Source: CAD feature listing. Evaluate the final solid. Frame: model axes, mm. Face numbers are marked on the shaded views. A direction names the side the tool comes from. Give positions to 0.01 mm unless a question says otherwise; leave off trailing zeros. Loops run counter-clockwise (first coordinate to the right, second up) from the corner with the lowest first, then second, coordinate; pieces in that order, holes last. Notation, with made-up numbers: M 83,22.25 L 102,22.25 A23 cw 102,59.25 Z; hole C 85,10.5 d5. An arc over 180 degrees is marked long. Answer in a Markdown table with one row per item.
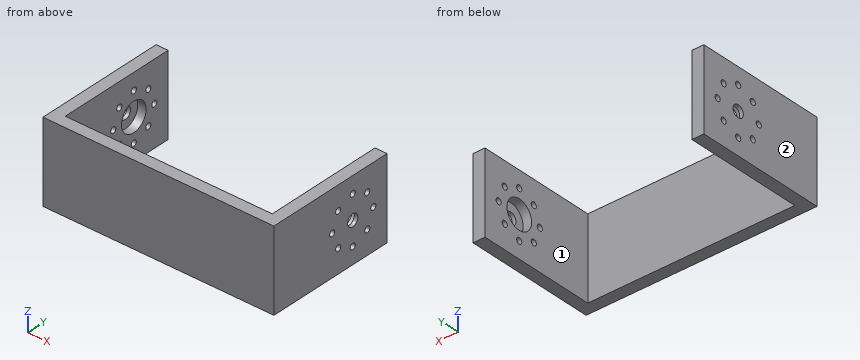
```python
from build123d import *

# Parameters (mm, degrees)
SKETCH1_W               = 57.8
SKETCH1_H               = 20.3
YAWMOUNT_DEPTH          = 3
SKETCH2_W               = 3
SKETCH2_H               = 20.3
BODYCONNECTORS_DEPTH    = 30
AXLE_MOUNTS_REACH       = 71.584
SKETCH3_R               = 1.5
SKETCH3_R_2             = 0.75
SKETCH4_R               = 3.6
SLIDE_COUNTERBORE_DEPTH = 2.12
GEAR_COUNTERBORE_START  = -2.1
SKETCH5_R               = 3.6
GEAR_COUNTERBORE_DEPTH  = 2.1


with BuildPart() as part:
    # Sketch1 → YawMount (new body)
    with BuildSketch(Plane(origin=(0, 0, 0), x_dir=(1, 0, 0), z_dir=(0, 1, 0))):
        with Locations((28.9, 10.15)):
            Rectangle(SKETCH1_W, SKETCH1_H)
    extrude(amount=YAWMOUNT_DEPTH)

    # Sketch2 → BodyConnectors (add)
    with BuildSketch(Plane(origin=(0, 3, 0), x_dir=(1, 0, 0), z_dir=(0, 1, 0))):
        with Locations((1.5, 10.15)):
            Rectangle(SKETCH2_W, SKETCH2_H)
        with Locations((56.3, 10.15)):
            Rectangle(SKETCH2_W, SKETCH2_H)
    extrude(amount=BODYCONNECTORS_DEPTH)

    # Axle-Mounts: up to this face of the body (flat: up to its plane)
    axle_mounts_end = Plane(part.part.faces().sort_by_distance((0, 16.5, -10.15))[0])
    # Sketch3 → Axle-Mounts (cut, up to the picked face)
    with BuildSketch(Plane(origin=(57.8, 0, 0), x_dir=(0, 0, -1), z_dir=(1, 0, 0)), mode=Mode.PRIVATE) as axle_mounts_sk1:
        with Locations((10.15, 23)):
            Circle(SKETCH3_R)
    axle_mounts_tool1 = split(extrude(axle_mounts_sk1.sketch, amount=-AXLE_MOUNTS_REACH, mode=Mode.PRIVATE), bisect_by=axle_mounts_end, keep=Keep.BOTH, mode=Mode.PRIVATE)
    # Sketch3 → Axle-Mounts (cut, up to the picked face)
    with BuildSketch(Plane(origin=(57.8, 0, 0), x_dir=(0, 0, -1), z_dir=(1, 0, 0)), mode=Mode.PRIVATE) as axle_mounts_sk2:
        with Locations((16.15, 23)):
            Circle(SKETCH3_R_2)
    axle_mounts_tool2 = split(extrude(axle_mounts_sk2.sketch, amount=-AXLE_MOUNTS_REACH, mode=Mode.PRIVATE), bisect_by=axle_mounts_end, keep=Keep.BOTH, mode=Mode.PRIVATE)
    # Sketch3 → Axle-Mounts (cut, up to the picked face)
    with BuildSketch(Plane(origin=(57.8, 0, 0), x_dir=(0, 0, -1), z_dir=(1, 0, 0)), mode=Mode.PRIVATE) as axle_mounts_sk3:
        with Locations((14.392640687, 18.757359313)):
            Circle(SKETCH3_R_2)
    axle_mounts_tool3 = split(extrude(axle_mounts_sk3.sketch, amount=-AXLE_MOUNTS_REACH, mode=Mode.PRIVATE), bisect_by=axle_mounts_end, keep=Keep.BOTH, mode=Mode.PRIVATE)
    # Sketch3 → Axle-Mounts (cut, up to the picked face)
    with BuildSketch(Plane(origin=(57.8, 0, 0), x_dir=(0, 0, -1), z_dir=(1, 0, 0)), mode=Mode.PRIVATE) as axle_mounts_sk4:
        with Locations((10.15, 17)):
            Circle(SKETCH3_R_2)
    axle_mounts_tool4 = split(extrude(axle_mounts_sk4.sketch, amount=-AXLE_MOUNTS_REACH, mode=Mode.PRIVATE), bisect_by=axle_mounts_end, keep=Keep.BOTH, mode=Mode.PRIVATE)
    # Sketch3 → Axle-Mounts (cut, up to the picked face)
    with BuildSketch(Plane(origin=(57.8, 0, 0), x_dir=(0, 0, -1), z_dir=(1, 0, 0)), mode=Mode.PRIVATE) as axle_mounts_sk5:
        with Locations((5.907359313, 18.757359313)):
            Circle(SKETCH3_R_2)
    axle_mounts_tool5 = split(extrude(axle_mounts_sk5.sketch, amount=-AXLE_MOUNTS_REACH, mode=Mode.PRIVATE), bisect_by=axle_mounts_end, keep=Keep.BOTH, mode=Mode.PRIVATE)
    # Sketch3 → Axle-Mounts (cut, up to the picked face)
    with BuildSketch(Plane(origin=(57.8, 0, 0), x_dir=(0, 0, -1), z_dir=(1, 0, 0)), mode=Mode.PRIVATE) as axle_mounts_sk6:
        with Locations((4.15, 23)):
            Circle(SKETCH3_R_2)
    axle_mounts_tool6 = split(extrude(axle_mounts_sk6.sketch, amount=-AXLE_MOUNTS_REACH, mode=Mode.PRIVATE), bisect_by=axle_mounts_end, keep=Keep.BOTH, mode=Mode.PRIVATE)
    # Sketch3 → Axle-Mounts (cut, up to the picked face)
    with BuildSketch(Plane(origin=(57.8, 0, 0), x_dir=(0, 0, -1), z_dir=(1, 0, 0)), mode=Mode.PRIVATE) as axle_mounts_sk7:
        with Locations((5.907359313, 27.242640687)):
            Circle(SKETCH3_R_2)
    axle_mounts_tool7 = split(extrude(axle_mounts_sk7.sketch, amount=-AXLE_MOUNTS_REACH, mode=Mode.PRIVATE), bisect_by=axle_mounts_end, keep=Keep.BOTH, mode=Mode.PRIVATE)
    # Sketch3 → Axle-Mounts (cut, up to the picked face)
    with BuildSketch(Plane(origin=(57.8, 0, 0), x_dir=(0, 0, -1), z_dir=(1, 0, 0)), mode=Mode.PRIVATE) as axle_mounts_sk8:
        with Locations((10.15, 29)):
            Circle(SKETCH3_R_2)
    axle_mounts_tool8 = split(extrude(axle_mounts_sk8.sketch, amount=-AXLE_MOUNTS_REACH, mode=Mode.PRIVATE), bisect_by=axle_mounts_end, keep=Keep.BOTH, mode=Mode.PRIVATE)
    # Sketch3 → Axle-Mounts (cut, up to the picked face)
    with BuildSketch(Plane(origin=(57.8, 0, 0), x_dir=(0, 0, -1), z_dir=(1, 0, 0)), mode=Mode.PRIVATE) as axle_mounts_sk9:
        with Locations((14.392640687, 27.242640687)):
            Circle(SKETCH3_R_2)
    axle_mounts_tool9 = split(extrude(axle_mounts_sk9.sketch, amount=-AXLE_MOUNTS_REACH, mode=Mode.PRIVATE), bisect_by=axle_mounts_end, keep=Keep.BOTH, mode=Mode.PRIVATE)
    add(axle_mounts_tool1.solids().sort_by(Axis((57.8, 23, -10.15), (-1, 0, 0)))[0], mode=Mode.SUBTRACT)
    add(axle_mounts_tool2.solids().sort_by(Axis((57.8, 23, -16.15), (-1, 0, 0)))[0], mode=Mode.SUBTRACT)
    add(axle_mounts_tool3.solids().sort_by(Axis((57.8, 18.757359, -14.392641), (-1, 0, 0)))[0], mode=Mode.SUBTRACT)
    add(axle_mounts_tool4.solids().sort_by(Axis((57.8, 17, -10.15), (-1, 0, 0)))[0], mode=Mode.SUBTRACT)
    add(axle_mounts_tool5.solids().sort_by(Axis((57.8, 18.757359, -5.907359), (-1, 0, 0)))[0], mode=Mode.SUBTRACT)
    add(axle_mounts_tool6.solids().sort_by(Axis((57.8, 23, -4.15), (-1, 0, 0)))[0], mode=Mode.SUBTRACT)
    add(axle_mounts_tool7.solids().sort_by(Axis((57.8, 27.242641, -5.907359), (-1, 0, 0)))[0], mode=Mode.SUBTRACT)
    add(axle_mounts_tool8.solids().sort_by(Axis((57.8, 29, -10.15), (-1, 0, 0)))[0], mode=Mode.SUBTRACT)
    add(axle_mounts_tool9.solids().sort_by(Axis((57.8, 27.242641, -14.392641), (-1, 0, 0)))[0], mode=Mode.SUBTRACT)

    # Sketch4 → Slide-Counterbore (cut)
    with BuildSketch(Plane.ZY.offset(-54.8)):
        with Locations((-10.15, 23)):
            Circle(SKETCH4_R)
    extrude(amount=-SLIDE_COUNTERBORE_DEPTH, mode=Mode.SUBTRACT)

    # Sketch5 → Gear-Counterbore (cut)
    with BuildSketch(Plane(origin=(3, 0, 0), x_dir=(0, 0, -1), z_dir=(1, 0, 0)).offset(GEAR_COUNTERBORE_START)):
        with Locations(Location((10.15, 23, 0), (0, 0, 180))):
            Circle(SKETCH5_R)
    extrude(amount=GEAR_COUNTERBORE_DEPTH, mode=Mode.SUBTRACT)


solid = part.part
```
1) Pin query (flat end, axial travel): pin 1 Ø10 at (x, z) = (16.5, -4.5) entering from +Y. Return the tip coordinate at first contact, or that it passes through.
Reply:
| item | result |
|---|---|
| pin 1 | stops at y = 3 |
2) Material intervals for L1, parallel to Y at x = 0.75, z = -10.15; L2, parallel to X at y = 24.5, z = -15.5; L3, parallel to X at y = 21, z = -7.25, sorted ascending.
Reply:
| item | result |
|---|---|
| L1 | y = 0 to 16.25, 17.75 to 21.5, 24.5 to 28.25, 29.75 to 33 |
| L2 | x = 0 to 3, 54.8 to 57.8 |
| L3 | x = 0 to 0.9, 56.92 to 57.8 |
3) Section C-C, the plane z = -4.15. Return loops of the section in (x, y), then the cut area to 3 significant figures.
Reply:
| item | result |
|---|---|
| outline | M 0,0 L 57.8,0 L 57.8,22.25 L 54.8,22.25 L 54.8,3 L 3,3 L 3,22.25 L 0,22.25 Z; M 0,23.75 L 3,23.75 L 3,33 L 0,33 Z; M 54.8,23.75 L 57.8,23.75 L 57.8,33 L 54.8,33 Z |
| area | 344 mm² |
4) Section B-B, the plane y = 31. Return loops of the section in (x, z), then the cut area to 3 significant figures.
Reply:
| item | result |
|---|---|
| outline | M 0,-20.3 L 3,-20.3 L 3,0 L 0,0 Z; M 54.8,-20.3 L 57.8,-20.3 L 57.8,0 L 54.8,0 Z |
| area | 122 mm² |
5) Section A-A, the plane y = 17. Return loops of the section in (x, z).
Reply:
| item | result |
|---|---|
| outline | M 0,-20.3 L 3,-20.3 L 3,-10.9 L 0,-10.9 Z; M 0,-9.4 L 3,-9.4 L 3,0 L 0,0 Z; M 54.8,-20.3 L 57.8,-20.3 L 57.8,-10.9 L 54.8,-10.9 Z; M 54.8,-9.4 L 57.8,-9.4 L 57.8,0 L 54.8,0 Z |
6) Section D-D, the plane z = -17.5. Return loops of the section in (x, y), then the cut area to 3 significant figures.
Reply:
| item | result |
|---|---|
| outline | M 0,0 L 57.8,0 L 57.8,33 L 54.8,33 L 54.8,3 L 3,3 L 3,33 L 0,33 Z |
| area | 353 mm² |
7) Set-up query: the marked faces 1 and 2. Return all of +Z, -Z, +X, -X, +Y, -Y with unobstructed straight access to the full face (end or side cutting, diameter ignored); none if empty.
Reply:
| item | result |
|---|---|
| face 1 | +Z, -Z, +Y |
| face 2 | +Z, -Z, -X, +Y, -Y |
